from build123d import *

# Parameters (mm, degrees)
SKETCH1_R               = 7
BOSS_EXTRUDE1_DEPTH     = 2
SKETCH2_R               = 3.98
CUT_EXTRUDE1_DEPTH      = 3
CUT_EXTRUDE1_DEPTH_BACK = 3
CUT_EXTRUDE2_START      = 2
SKETCH3_R               = 6.12
SKETCH3_R_2             = 4.9
CUT_EXTRUDE2_DEPTH      = 0.2


with BuildPart() as part:
    # Sketch1 → Boss-Extrude1 (new body, symmetric)
    with BuildSketch(Plane(origin=(0, 0, 0), x_dir=(1, 0, 0), z_dir=(0, 1, 0))):
        Circle(SKETCH1_R)
    extrude(amount=BOSS_EXTRUDE1_DEPTH, both=True)

    # Sketch2 → Cut-Extrude1 (cut, two sides)
    with BuildSketch(Plane(origin=(0, 0, 0), x_dir=(1, 0, 0), z_dir=(0, 1, 0))) as cut_extrude1_sk:
        Circle(SKETCH2_R)
    extrude(amount=CUT_EXTRUDE1_DEPTH, mode=Mode.SUBTRACT)
    extrude(cut_extrude1_sk.sketch, amount=-CUT_EXTRUDE1_DEPTH_BACK, mode=Mode.SUBTRACT)

    # Sketch3 → Cut-Extrude2 (cut)
    with BuildSketch(Plane(origin=(0, 0, 0), x_dir=(1, 0, 0), z_dir=(0, 1, 0)).offset(CUT_EXTRUDE2_START)):
        Circle(SKETCH3_R)
        Circle(SKETCH3_R_2, mode=Mode.SUBTRACT)
    cut_extrude2 = extrude(amount=-CUT_EXTRUDE2_DEPTH, mode=Mode.SUBTRACT)

    # Mirror1: Cut-Extrude2 across plane
    add(cut_extrude2.mirror(Plane.ZX), mode=Mode.SUBTRACT)


solid = part.part
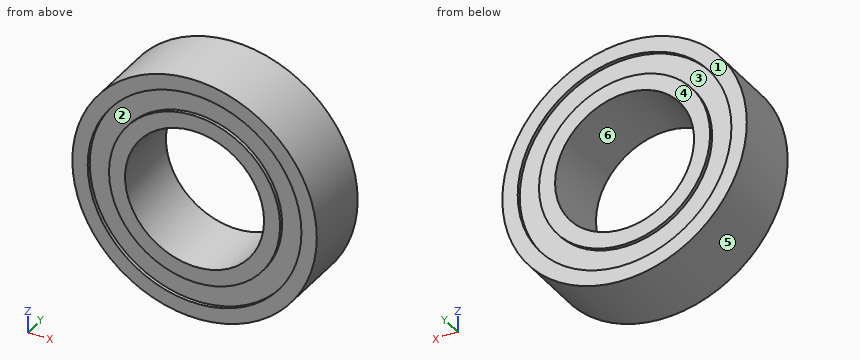
Geometry: final body of the model. Coordinates: model frame, mm. Face numbers are marked on the shaded views. A direction names the side the tool comes from. Give positions to 0.01 mm unless a question says otherwise; leave off trailing zeros. Write each loop counter-clockwise with the first axis right and the second up, starting at its lowest first coordinate (ties: lowest second). Pieces come first, ordered by that corner, then holes.
(1) First-contact query: P1, Ø2, axis at x = 2.5, y = -1, coming from the -Z side; P2, Ø1, axis at x = 1, y = 1.5, coming from the +Z side; P3, Ø1.5, axis at x = -4.5, y = -1, coming from the -Z side. Flat tips, straight axial feed; report the tip coordinate or a pass-through.
(2) Ray query, line 1 (Z direction, x = 0, y = -1.85); line 2 (Z direction, x = 0, y = -0.35). Return the intervals inside material, ascending.
(3) Cut plane D-D, the plane z = 5.5. Return loops of the section in (x, y), then the cut area to 3 significant figures.
(4) Cut plane B-B, the plane x = 0. Return loops of the section in (y, z).
(5) Cut plane C-C, the plane y = 0.05. Return loops of the section in (x, z).
(6) Cut plane A-A, the plane z = 0. Return loops of the section in (x, y).
(7) Access query for the marked faces 1, 2 and 3. Directions: +Z, -Z, +X, -X, +Y, -Y. A direction counts if a zero-diameter tool reaches every point of the face in a straight line with its end or side. Return the directions, or none.
(8) Mould query, pull axis Z, two halves, no side actions, for the marked faces 4, 5 and 6. Classes: released by +Z, released by -Z, zero draft, split by the parting line, or undercut.
Values follow:
1. P1: stops at z = -6.84
1. P2: stops at z = 6.98
1. P3: stops at z = -5.91
2. line 1: z = -7 to -6.12, -4.9 to -3.98, 3.98 to 4.9, 6.12 to 7
2. line 2: z = -7 to -3.98, 3.98 to 7
3. outline: (-4.33, -2) - (-2.68, -2) - (-2.68, -1.8) - (2.68, -1.8) - (2.68, -2) - (4.33, -2) - (4.33, 2) - (2.68, 2) - (2.68, 1.8) - (-2.68, 1.8) - (-2.68, 2) - (-4.33, 2) - close
3. area: 32.5 mm2
4. outline: (-2, -7) - (2, -7) - (2, -6.12) - (1.8, -6.12) - (1.8, -4.9) - (2, -4.9) - (2, -3.98) - (-2, -3.98) - (-2, -4.9) - (-1.8, -4.9) - (-1.8, -6.12) - (-2, -6.12) - close; (-2, 3.98) - (2, 3.98) - (2, 4.9) - (1.8, 4.9) - (1.8, 6.12) - (2, 6.12) - (2, 7) - (-2, 7) - (-2, 6.12) - (-1.8, 6.12) - (-1.8, 4.9) - (-2, 4.9) - close
5. outline: circle Ø14 at (0, 0); hole circle Ø7.96 at (0, 0)
6. outline: (-7, -2) - (-6.12, -2) - (-6.12, -1.8) - (-4.9, -1.8) - (-4.9, -2) - (-3.98, -2) - (-3.98, 2) - (-4.9, 2) - (-4.9, 1.8) - (-6.12, 1.8) - (-6.12, 2) - (-7, 2) - close; (3.98, -2) - (4.9, -2) - (4.9, -1.8) - (6.12, -1.8) - (6.12, -2) - (7, -2) - (7, 2) - (6.12, 2) - (6.12, 1.8) - (4.9, 1.8) - (4.9, 2) - (3.98, 2) - close
7. face 1: +Z, -Z, +X, -X, +Y
7. face 2: -Y
7. face 3: +Y
8. face 4: zero draft
8. face 5: split by the parting line
8. face 6: undercut
